from build123d import *

# Parameters (mm, degrees)
SKETCH1_R           = 5
BOSS_EXTRUDE1_DEPTH = 5


with BuildPart() as part:
    # Sketch1 → Boss-Extrude1 (new, symmetric)
    with BuildSketch(Plane.XY):
        with BuildLine():
            ThreePointArc((-14.999916666, -0.05), (0, -15), (14.999916666, -0.05))
            ThreePointArc((14.999916666, -0.05), (12.474592102, 17.374981858), (4.999972222, 33.316666667))
            ThreePointArc((4.999972222, 33.316666667), (0, 36), (-4.999972222, 33.316666667))
            ThreePointArc((-4.999972222, 33.316666667), (-12.474592102, 17.374981858), (-14.999916666, -0.05))
        make_face()
        Circle(SKETCH1_R, mode=Mode.SUBTRACT)
    extrude(amount=BOSS_EXTRUDE1_DEPTH, both=True)


solid = part.part
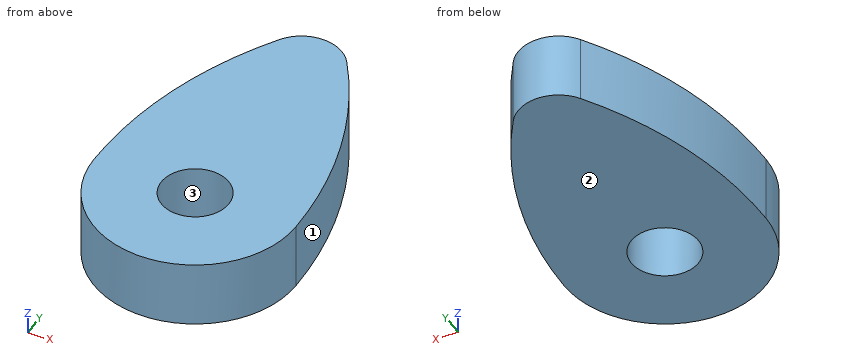
Verification items for the finished model (mm, model axes). Face numbers are marked on the shaded views. Give positions to 0.01 mm unless a question says otherwise; leave off trailing zeros. Loops run counter-clockwise (first coordinate to the right, second up) from the corner with the lowest first, then second, coordinate; pieces in that order, holes last.
1) Depth check by flat-ended pin: pin 1 Ø9 at (x, y) = (0, 0) entering from -Z; pin 2 Ø1 at (x, z) = (3.5, 4) entering from -Y; pin 3 Ø1.5 at (x, z) = (3, -1) entering from -Y; pin 4 Ø2 at (x, z) = (8, 1.5) entering from +Y. Enter the tip coordinate at first touch or a pass-through.
2) Sectioned sample at B-B, the plane z = -2. Enter the section's corners in (x, y).
3) Sectioned sample at A-A, the plane x = 0. Enter the section's corners in (y, z), then the cut area to 3 significant figures.
4) Thickness scan on line 1 along Y through (x, z) = (0, -3); line 2 along X through (y, z) = (26, 0); line 3 along X through (y, z) = (23, -4). Record the ranges inside material, lowest first.
5) Draft check along X on the marked faces 1, 2 and 3. Enter one of: pulls with the +X half, pulls with the -X half, needs draft (parallel to the pull), parting line crosses it, or undercut.
6) Sectioned sample at C-C, the plane x = -12. Enter the section's corners in (y, z), then the cut area to 3 significant figures.
7) Sectioned sample at D-D, the plane y = 15. Enter the section's corners in (x, z).
Answers:
1. pin 1: passes through
1. pin 2: stops at y = -14.7
1. pin 3: stops at y = -14.83
1. pin 4: stops at y = 30.08
2. outline: (-15, -0.05) arc R15 ccw to (15, -0.05) arc R60 ccw to (5, 33.32) arc R6 ccw to (-5, 33.32) arc R60 ccw to start; hole circle Ø10 at (0, 0)
3. outline: (-15, -5) - (-5, -5) - (-5, 5) - (-15, 5) - close; (5, -5) - (36, -5) - (36, 5) - (5, 5) - close
3. area: 410 mm2
4. line 1: y = -15 to -5, 5 to 36
4. line 2: x = -9.15 to 9.15
4. line 3: x = -10.48 to 10.48
5. face 1: pulls with the +X half
5. face 2: needs draft
5. face 3: undercut
6. outline: (-9, -5) - (18.89, -5) - (18.89, 5) - (-9, 5) - close
6. area: 279 mm2
7. outline: (-13.13, -5) - (13.13, -5) - (13.13, 5) - (-13.13, 5) - close
